```python
from build123d import *

# Parameters (mm, degrees)
SKETCH1_R           = 36.785134715
BOSS_EXTRUDE1_DEPTH = 3.683
SKETCH2_R           = 1.8415


with BuildPart() as part:
    # Sketch1 → Boss-Extrude1 (new body)
    with BuildSketch(Plane(origin=(0, 0, 0), x_dir=(1, 0, 0), z_dir=(0, 1, 0))):
        with Locations(Location((0, 0, 0), (0, 0, 270))):
            Circle(SKETCH1_R)
        with BuildLine():
            Line((-1.099852263, 32.146289174), (-13.115875302, 11.333926765))
            ThreePointArc((-13.115875302, 11.333926765), (-13.242748838, 10.370226578), (-12.651023039, 9.599074503))
            Line((-12.651023039, 9.599074503), (-7.368281269, 6.549082119))
            ThreePointArc((-7.368281269, 6.549082119), (-8.559992893, 4.889638753), (-9.384056343, 3.020187413))
            Line((-9.384056343, 3.020187413), (-14.683023039, 6.079547262))
            ThreePointArc((-14.683023039, 6.079547262), (-15.646723226, 6.206420798), (-16.417875302, 5.614694999))
            Line((-16.417875302, 5.614694999), (-28.389429193, -15.120644587))
            ThreePointArc((-28.389429193, -15.120644587), (-28.389429193, -16.390644587), (-27.289576931, -17.025644587))
            Line((-27.289576931, -17.025644587), (-3.302, -17.025644587))
            ThreePointArc((-3.302, -17.025644587), (-2.403974388, -16.653670199), (-2.032, -15.755644587))
            Line((-2.032, -15.755644587), (-2.032, -9.646399404))
            ThreePointArc((-2.032, -9.646399404), (0, -9.858095427), (2.032, -9.646399404))
            Line((2.032, -9.646399404), (2.032, -15.755644587))
            ThreePointArc((2.032, -15.755644587), (2.403974388, -16.653670199), (3.302, -17.025644587))
            Line((3.302, -17.025644587), (27.289576931, -17.025644587))
            ThreePointArc((27.289576931, -17.025644587), (28.389429193, -16.390644587), (28.389429193, -15.120644587))
            Line((28.389429193, -15.120644587), (16.395640728, 5.65320641))
            ThreePointArc((16.395640728, 5.65320641), (15.624488653, 6.24493221), (14.660788465, 6.118058673))
            Line((14.660788465, 6.118058673), (9.370026939, 3.063436081))
            ThreePointArc((9.370026939, 3.063436081), (8.537361073, 4.929047714), (7.338026939, 6.582963322))
            Line((7.338026939, 6.582963322), (12.628788465, 9.637585914))
            ThreePointArc((12.628788465, 9.637585914), (13.220514265, 10.408737989), (13.093640728, 11.372438177))
            Line((13.093640728, 11.372438177), (1.099852263, 32.146289174))
            ThreePointArc((1.099852263, 32.146289174), (0, 32.781289174), (-1.099852263, 32.146289174))
        make_face(mode=Mode.SUBTRACT)
        with BuildLine():
            Line((-2.693461931, 31.926076262), (-28.995524051, -13.630431675))
            ThreePointArc((-28.995524051, -13.630431675), (-30.168979582, -14.26329703), (-31.261319719, -13.498895652))
            ThreePointArc((-31.261319719, -13.498895652), (-29.489281456, 17.025644587), (-3.940273302, 33.822544859))
            ThreePointArc((-3.940273302, 33.822544859), (-2.732112221, 33.258751239), (-2.693461931, 31.926076262))
        make_face(mode=Mode.SUBTRACT)
        with BuildLine():
            Line((2.693461931, 31.926076262), (28.995524051, -13.630431675))
            ThreePointArc((28.995524051, -13.630431675), (30.168979582, -14.26329703), (31.261319719, -13.498895652))
            ThreePointArc((31.261319719, -13.498895652), (29.489281456, 17.025644587), (3.940273302, 33.822544859))
            ThreePointArc((3.940273302, 33.822544859), (2.732112221, 33.258751239), (2.693461931, 31.926076262))
        make_face(mode=Mode.SUBTRACT)
        with BuildLine():
            Line((-26.302062121, -18.295644587), (26.302062121, -18.295644587))
            ThreePointArc((26.302062121, -18.295644587), (27.436867361, -18.995454209), (27.321046417, -20.323649206))
            ThreePointArc((27.321046417, -20.323649206), (0, -34.051289174), (-27.321046417, -20.323649206))
            ThreePointArc((-27.321046417, -20.323649206), (-27.436867361, -18.995454209), (-26.302062121, -18.295644587))
        make_face(mode=Mode.SUBTRACT)
    extrude(amount=BOSS_EXTRUDE1_DEPTH)

    # Sketch2 → Cut-Revolve2 (revolve, cut)
    with BuildSketch(Plane.XY, mode=Mode.PRIVATE) as cut_revolve2_sk:
        with Locations((36.785134715, 1.8415)):
            Circle(SKETCH2_R)
    revolve(cut_revolve2_sk.sketch.rotate(Axis((0, 0, 0), (0, 1, 0)), 90), axis=Axis((0, 0, 0), (0, 1, 0)), mode=Mode.SUBTRACT)


solid = part.part
```
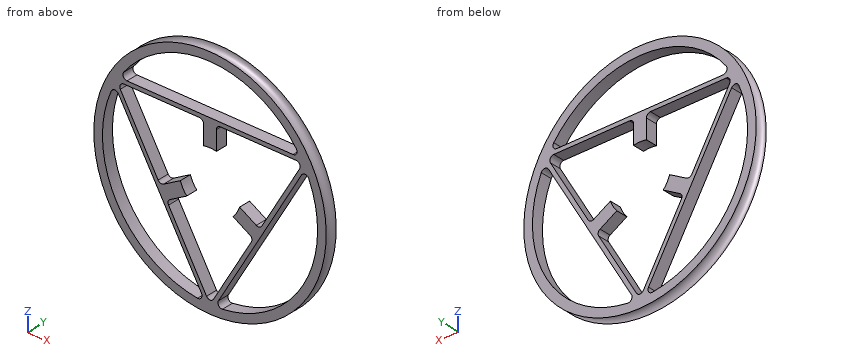
The model under review builds one solid part; all positions refer to its coordinate system, in mm. Round coordinates to 2 decimals unless told otherwise and drop trailing zeros. Write item = value, one per line.
Item 1: Take a section at A-A on z = -21.5. State how many separate pieces and enclosed holes the cut face has, then the cut area to 3 significant figures.
Return value:
separate_pieces = 4
enclosed_holes = 0
area = 22.9 mm2
Item 2: For line 1 (Z direction, x = 26, y = 2.05); line 2 (Z direction, x = 16.5, y = 1.1); line 3 (Z direction, x = -7.5, y = 3.1), list the stretches that pass through material, from the lowest coordinate up. Write a range as [from, to].
Return value:
line_1 = [-23.36, -21.99], [8.44, 10.98], [17.03, 18.3], [21.99, 23.36]
line_2 = [-30.98, -29.79], [-8.01, -5.47], [17.03, 18.3], [29.79, 30.98]
line_3 = [-34.64, -33.22], [-23.6, -21.06], [-6.63, -6.4], [17.03, 18.3], [33.22, 34.64]
Item 3: Insertion check: P1, Ø3, axis at x = -23.5, z = 11, coming from the +Y side; P2, Ø1.1, axis at x = -18, y = 1, coming from the -Z side; P3, Ø1.8, axis at x = 12, y = 2, coming from the -Z side; P4, Ø1, axis at x = -23.5, y = 1.5, coming from the +Z side. Each pin has a flat end and moves straight along its axis. Give the tip position at first contact, or say it passes through.
Return value:
P1 = through
P2 = -30.76
P3 = -33.25
P4 = 26.38
